Geometry check sheet. Reference: the model listing, model coordinates, mm. A direction names the side the tool comes from. Round coordinates to 2 decimals unless told otherwise and drop trailing zeros. Order: outer loops, then holes, each group sorted by start corner. A loop starts at its lowest first (then second) coordinate and runs counter-clockwise, first axis right, second up.
Autodesk Inventor part; units mm, degrees
ref_plane "Lifted XZ Plane" through (0, 45, 0) normal (0, -1, 0) x (1, 0, 0)
ref_plane "YZ Plane" through (0, 0, 0) normal (1, 0, 0) x (0, 1, 0)
ref_plane "XZ Plane" through (0, 0, 0) normal (0, 1, 0) x (-1, 0, 0)
sketch "Main Sketch" plane through (0, 0, 0) normal (0, 1, 0) x (-1, 0, 0)
  line L0 (-57.375, -12.0472) -> (-57.375, 12.0472)
  line L1 (-57.375, 12.0472) -> (47.625, -10) construction
  line L2 (47.625, 10) -> (-57.375, -12.0472) construction
  circle A0 centre (47.625, 0) radius 7
  arc A1 (47.625, -10) -> (47.625, 10) centre (47.625, 0) ccw
  line L3 (-40.875, 17.5) -> (-57.375, 17.5)
  line L4 (-57.375, 17.5) -> (-57.375, -17.5)
  line L5 (-57.375, -17.5) -> (-40.875, -17.5)
  line L6 (-40.875, 17.5) -> (-57.375, -17.5) construction
  line L7 (-57.375, 17.5) -> (-40.875, -17.5) construction
  line L8 (47.625, -10) -> (-40.875, -10)
  line L9 (-40.875, -17.5) -> (-40.875, -10)
  line L10 (-40.875, 10) -> (-40.875, 17.5)
  line L11 (-40.875, 10) -> (47.625, 10)
  point P0 (0, 0)
  point P1 (-49.125, 0)
  dimension "d3" = 14
  dimension "d4" = 105
  dimension "d13" = 16.5
  dimension "d14" = 35
  dimension "d15" = 0
  dimension "d18" = 20
extrude "Main Extrusion" add sketch "Main Sketch" along normal blind 4
sketch "Screw Holes Sketch" plane through (0, 4, 0) normal (0, 1, 0) x (1, 0, 0)
  circle A0 centre (46.125, -8.75) radius 2
  line L0 (57.375, 17.5) -> (40.875, 17.5)
  line L1 (40.875, -17.5) -> (57.375, -17.5)
  line L2 (35.2664, 0) -> (65.7891, 0)
  line L3 (51.375, -27.0398) -> (51.375, 30.2346) construction
  line L4 (57.375, -17.5) -> (57.375, 17.5)
  line L5 (40.875, -10) -> (40.875, -17.5)
  circle A1 centre (46.125, 8.75) radius 2
  line L6 (51.375, 27.0398) -> (51.375, -30.2346) construction
  point P0 (0, 0)
  dimension "d21" = 4
  dimension "d22" = 35
  dimension "d23" = 6
  dimension "d24" = 5.25
  dimension "d25" = 5.25
  dimension "d26" = 10.5
  dimension "d27" = 8.75
  dimension "d28" = 17.5
extrude "Screw Holes Cut" cut sketch "Screw Holes Sketch" against normal through all
fillet "Smoooooooooooooooooth" radius 6 2 edges at (40.875, 2, -17.5) (40.875, 2, 17.5)
sketch "Side Axel Hole Sketch" plane through (-47.625, 0, 10) normal (0, 0, 1) x (1, 0, 0)
  line L0 (88.5, 4) -> (88.5, 0)
  line L1 (0, 0) -> (0, 4)
  line L2 (44.25, -12.0383) -> (44.25, 22.7681) construction
  line L3 (88.5, 0) -> (0, 0)
  line L4 (0, 4) -> (88.5, 4)
  circle A0 centre (44.25, 4) radius 1.5
  point P0 (47.625, 0)
  dimension "d32" = 88.5
  dimension "d33" = 44.25
  dimension "d34" = 44.25
  dimension "d35" = 4
  dimension "d41" = 3
sketch "Sketch7" plane through (0, 4, 0) normal (0, 1, 0) x (1, 0, 0)
  line L0 (-47.625, -10) -> (40.875, -10) construction
  line L1 (-3.375, -10) -> (-3.375, 33.3565) construction
  line L2 (-0.3194, -13) -> (-6.4306, -13)
  line L3 (-6.4306, -13) -> (-6.4306, 13)
  line L4 (-6.4306, 13) -> (-0.3194, 13)
  line L5 (-0.3194, 13) -> (-0.3194, -13)
  line L6 (-0.3194, -13) -> (-6.4306, 13) construction
  line L7 (-6.4306, -13) -> (-0.3194, 13) construction
  point P0 (0, 0)
  point P1 (-3.375, 0)
  dimension "d47" = 26
extrude "Servo Mount Extrusion" add sketch "Sketch7" along normal blind 62.8 and the other way blind 4
extrude "Side Axel Cut" cut sketch "Side Axel Hole Sketch" along normal through all both and the other way through all contours A0 L4 | L4 A0
sketch "Sketch8" plane through (-6.4306, 4, -10) normal (-1, 0, 0) x (0, 0, 1)
  line L0 (23, 62.8) -> (23, -4) construction
  line L1 (-3, 62.8) -> (23, 62.8) construction
  line L2 (-3, 62.8) -> (-3, -4) construction
  circle A0 centre (2, 55.8) radius 2
  circle A1 centre (18, 55.8) radius 2
  point P0 (10, -4)
  dimension "d54" = 4
  dimension "d55" = 4
  dimension "d56" = 16
  dimension "d57" = 7
  dimension "d58" = 7
  dimension "d59" = 5
  dimension "d60" = 5
extrude "Mount Holes Cut" cut sketch "Sketch8" against normal through all
fillet "Support" radius 41 1 edges at (-0.3194, 4, 0)
fillet "lil hat" radius 3 4 edges at (-0.3194, 66.8, 0) (-3.375, 66.8, -13) (-6.4306, 66.8, 0) (-3.375, 66.8, 13)
ref_plane "Lifted XZ Plane" through (0, 45, 0) normal (0, -1, 0) x (1, 0, 0)
sketch "Support Center Sketch" plane through (0, 45, 0) normal (0, -1, 0) x (1, 0, 0)
  line L0 (40.6806, 10) -> (40.6806, -10)
  line L1 (-0.3194, -6) -> (40.6806, -6)
  line L2 (40.6806, -6) -> (40.6806, 6)
  line L3 (40.6806, 6) -> (-0.3194, 6)
  line L4 (-0.3194, 6) -> (-0.3194, -6)
  line L5 (-0.3194, -10) -> (40.6806, -10)
  line L6 (40.6806, 10) -> (-0.3194, 10)
  point P0 (0, 0)
  dimension "d66" = 41
  dimension "d67" = 4
  dimension "d68" = 4
  dimension "d69" = 12
extrude "Support Center Cut" cut sketch "Support Center Sketch" along normal blind 41
sketch "Support Side Cut Sketch" plane through (40.875, 0, -10) normal (0, 0, -1) x (-1, 0, 0)
  arc A0 (0.1944, 4) -> (41.1944, 45) centre (0.1944, 45) ccw construction
  arc A1 (0.1944, 4) -> (41.1944, 45) centre (0.1944, 45) ccw
  arc A2 (18.7416, 4) -> (41.1944, 26.4528) centre (0.1944, 45) ccw
  line L0 (-6, 4) -> (0, 4)
  line L1 (41.1944, 0) -> (41.1944, 45)
  line L2 (41.1944, 0) -> (0, 0)
  line L3 (41.1944, 26.4528) -> (41.1944, 4)
  line L4 (0, 4) -> (0.1944, 4)
  line L5 (18.7416, 4) -> (41.1944, 4)
  point P0 (40.875, 0)
  dimension "d72" = 41
  dimension "d73" = 45
  dimension "d75" = 4
extrude "Support Side Cut" cut sketch "Support Side Cut Sketch" against normal through all
sketch "Body Holes Sketch" plane through (0, 4, 0) normal (0, 1, 0) x (1, 0, 0)
  line L0 (-37.625, 4) -> (-8.4306, 4)
  line L1 (-8.4306, 4) -> (-8.4306, 8)
  line L2 (-8.4306, 8) -> (-37.625, 8)
  line L3 (-37.625, 8) -> (-37.625, 4)
  line L4 (-6.4306, 10) -> (-47.625, 10)
  line L5 (-6.4306, -10) -> (-6.4306, 10)
  line L6 (-47.625, -13.767) -> (-47.625, 22.327) construction
  line L7 (-37.625, -2) -> (-8.4306, -2)
  line L8 (-8.4306, -2) -> (-8.4306, 2)
  line L9 (-8.4306, 2) -> (-37.625, 2)
  line L10 (-37.625, 2) -> (-37.625, -2)
  line L11 (-37.625, -8) -> (-8.4306, -8)
  line L12 (-8.4306, -8) -> (-8.4306, -4)
  line L13 (-8.4306, -4) -> (-37.625, -4)
  line L14 (-37.625, -4) -> (-37.625, -8)
  line L15 (-47.625, -10) -> (-6.4306, -10)
  line L16 (39.4306, 3) -> (1.6806, 3)
  line L17 (1.6806, 3) -> (1.6806, -3)
  line L18 (1.6806, -3) -> (39.4306, -3)
  line L19 (39.4306, -3) -> (39.4306, 3)
  line L20 (40.6806, -6) -> (-0.3194, -6)
  line L21 (-0.3194, 6) -> (40.6806, 6)
  line L22 (-0.3194, 10) -> (-0.3194, -10)
  line L23 (40.6806, 6) -> (40.6806, 10)
  point P0 (0, 0)
  dimension "d78" = 2
  dimension "d79" = 2
  dimension "d80" = 10
  dimension "d81" = 4
  dimension "d84" = 6
  dimension "d89" = 2
  dimension "d90" = 6
  dimension "d91" = 3
  dimension "d92" = 3
  dimension "d93" = 2
  dimension "d94" = 1.25
extrude "Swiss-ified" cut sketch "Body Holes Sketch" against normal through all
sketch "Mount Hole Sketch" plane through (-6.4306, 4, -10) normal (-1, 0, 0) x (0, 0, 1)
  line L0 (4, 81.3032) -> (4, -34.1238) construction
  line L1 (16, 81.3032) -> (16, -34.1238) construction
  line L2 (7, 3) -> (13, 3)
  line L3 (13, 3) -> (13, 57.8)
  line L4 (13, 57.8) -> (7, 57.8)
  line L5 (7, 57.8) -> (7, 3)
  line L6 (-3, 59.8) -> (-3, -4)
  line L7 (23, 59.8) -> (23, -4)
  line L8 (20, 0) -> (0, 0)
  line L9 (-3, 59.8) -> (23, 59.8)
  point P0 (10, -4)
  dimension "d97" = 6
  dimension "d98" = 7
  dimension "d99" = 7
  dimension "d100" = 12
  dimension "d101" = 3
  dimension "d102" = 3
  dimension "d103" = 3
  dimension "d104" = 2
extrude "Swissified" cut sketch "Mount Hole Sketch" against normal through all
properties part number "TapeMeasureBracketSideServo"
(1) Draft check along X on faces 5 (the flat face through (13, 0, 4)), 6 (the flat face through (-23, 2, 8)). Enter one of: released by +X, released by -X, zero draft, split by the parting line, or undercut.
Returned:
face 5: zero draft
face 6: undercut
(2) Sectioned sample at B-B, the plane y = 18.5. Record the cut outline in (x, z), and give its area (3 significant figures).
Returned:
outline: (-6.43, -13) - (-0.32, -13) - (-0.32, -3) - (-6.43, -3) - close; (-6.43, 3) - (-0.32, 3) - (-0.32, 13) - (-6.43, 13) - close; (4.31, -10) - (9.4, -10) - (9.4, -6) - (4.31, -6) - close; (4.31, 6) - (9.4, 6) - (9.4, 10) - (4.31, 10) - close
area: 163 mm2
(3) Sectioned sample at C-C, the plane y = 36.5. Record the cut outline in (x, z), and give its area (3 significant figures).
Returned:
outline: (-6.43, -13) - (-0.32, -13) - (-0.32, -10) - (0.57, -10) - (0.57, -6) - (-0.32, -6) - (-0.32, -3) - (-6.43, -3) - close; (-6.43, 3) - (-0.32, 3) - (-0.32, 6) - (0.57, 6) - (0.57, 10) - (-0.32, 10) - (-0.32, 13) - (-6.43, 13) - close
area: 129 mm2
(4) Material ranges on line 1 (Y direction, x = -4, z = 8); line 2 (Z direction, x = 26.5, y = 3); line 3 (Y direction, x = -14, z = -3), recorded low to high.
Returned:
line 1: y = 0 to 2.64, 5.36 to 57.8, 61.8 to 66.75
line 2: z = -10 to -3, 3 to 10
line 3: y = 0 to 4
(5) Set-up check for faces 1 (the flat face through (16, 9, 10)), 2 (the flat face through (-37.625, 2, 0)), 3 (the flat face through (-27, 2, 10)), 4 (the flat face through (35, 4, 4)): record each of +Z, -Z, +X, -X, +Y, -Y from which the full face is reachable in a straight line by a thin tool's end or side.
Returned:
face 1: +Z, +Y, -Y
face 2: +Y, -Y
face 3: +Z, -X, +Y, -Y
face 4: none
(6) Sectioned sample at D-D, the plane x = 29.5. Record the cut outline in (y, z).
Returned:
outline: (0, -10) - (5.55, -10) - (5.55, -6) - (4, -6) - (4, -3) - (0, -3) - close; (0, 3) - (4, 3) - (4, 6) - (5.55, 6) - (5.55, 10) - (0, 10) - close
(7) Depth check by flat-ended pin: P1, Ø0.8, axis at y = 2.5, z = -11, coming from the -X side; P2, Ø1.5, axis at y = 46.5, z = 13, coming from the +X side; P3, Ø1.2, axis at x = -18.5, y = 3, coming from the -Z side. Enter the tip coordinate at first touch or a pass-through.
Returned:
P1: stops at x = -6.43
P2: stops at x = -0.32
P3: stops at z = -10
(8) Sectioned sample at A-A, the plane x = -27.5. Record the cut outline in (y, z).
Returned:
outline: (0, -10) - (4, -10) - (4, -8) - (0, -8) - close; (0, -4) - (4, -4) - (4, -2) - (0, -2) - close; (0, 2) - (4, 2) - (4, 4) - (0, 4) - close; (0, 8) - (4, 8) - (4, 10) - (0, 10) - close
